Source: CAD feature listing. Evaluate the final solid. Frame: model axes, mm. Face numbers are marked on the shaded views. Coordinates: 2 decimals unless noted, no trailing zeros. Write each loop counter-clockwise with the first axis right and the second up, starting at its lowest first coordinate (ties: lowest second). Pieces come first, ordered by that corner, then holes. Notation, with made-up numbers: M 56,68.25 L 113,68.25 A15 cw 113,75.25 Z; hole C 33,-39.5 d11. An arc over 180 degrees is marked long. One line per item, written item: value. Start each with the question number.
Item 1: Mould query, pull axis Y, two halves, no side actions, for the marked faces 1 and 2. Classes: released by +Y, released by -Y, zero draft, split by the parting line, or undercut.
Item 2: Ray query, L1, parallel to Y at x = 73, z = 2.5; L2, parallel to Y at x = 50, z = 3.75; L3, parallel to Y at x = 81.5, z = 2. Return the intervals inside material, ascending. Write a range as from..to.
Item 3: Pin query (flat end, axial travel): P1, Ø1.5, axis at x = 123.5, z = 1.5, coming from the +Y side; P2, Ø5, axis at x = 86.035, y = -31.25, coming from the -Z side; P3, Ø20, axis at x = 59.509, y = 0, coming from the +Z side; P4, Ø4, axis at x = 39.549, y = 67.25, coming from the -Z side. Return the tip coordinate at first contact, or that it passes through.
Item 4: Cut plane A-A, the plane y = 0. Output: boundary loops of the cut face in (x, z), then the cut area to 3 significant figures.
Item 5: Cut plane D-D, the plane y = 40.5. Output: boundary loops of the cut face in (x, z), then the cut area to 3 significant figures.
Item 6: Cut plane C-C, the plane y = -23.5. Output: boundary loops of the cut face in (x, z), then the cut area to 3 significant figures.
Item 7: Cut plane B-B, the plane y = 67.25. Output: boundary loops of the cut face in (x, z).
Autodesk Inventor part; units mm, degrees
ref_plane "YZ Plane" through (0, 0, 0) normal (1, 0, 0) x (0, 1, 0)
ref_plane "XZ Plane" through (0, 0, 0) normal (0, 1, 0) x (-1, 0, 0)
ref_plane "XY Plane" through (0, 0, 0) normal (0, 0, 1) x (1, 0, 0)
sketch "Sketch1" plane through (0, 0, 0) normal (0, 0, 1) x (1, 0, 0)
  circle A0 centre (-11.3135, -11.3135) radius 2
  circle A1 centre (-11.3135, 11.3135) radius 2
  circle A2 centre (11.3135, 11.3135) radius 2
  circle A3 centre (11.3135, -11.3135) radius 2
  circle A4 centre (-15.3135, 11.3135) radius 2
  circle A5 centre (-7.3135, 11.3135) radius 2
  circle A6 centre (7.3135, 11.3135) radius 2
  circle A7 centre (15.3135, 11.3135) radius 2
  circle A8 centre (15.3135, -11.3135) radius 2
  circle A9 centre (7.3135, -11.3135) radius 2
  circle A10 centre (-7.3135, -11.3135) radius 2
  circle A11 centre (-15.3135, -11.3135) radius 2
  line L0 (-15.3135, 13.3135) -> (-7.3135, 13.3135)
  line L1 (-7.3135, 9.3135) -> (-15.3135, 9.3135)
  line L2 (-15.3135, -9.3135) -> (-7.3135, -9.3135)
  line L3 (-7.3135, -13.3135) -> (-15.3135, -13.3135)
  line L4 (7.3135, -9.3135) -> (15.3135, -9.3135)
  line L5 (15.3135, -13.3135) -> (7.3135, -13.3135)
  line L6 (15.3135, 9.3135) -> (7.3135, 9.3135)
  line L7 (15.3135, 13.3135) -> (7.3135, 13.3135)
  circle A12 centre (0, 0) radius 8.25
  circle A13 centre (5, 0) radius 8.25
  circle A14 centre (-5, 0) radius 8.25
  line L8 (-5, 8.25) -> (5, 8.25)
  line L9 (5, -8.25) -> (-5, -8.25)
  circle A15 centre (0, 0) radius 42.5
  circle A16 centre (59.509, 0) radius 50.7821
  line L10 (-5.9149, 42.0864) -> (52.4415, 50.2878)
  line L11 (-5.9149, -42.0864) -> (52.4415, -50.2878)
  line L12 (-13.25, 0) -> (13.25, 0)
  circle A17 centre (59.509, 0) radius 11
  arc A18 (-5.9149, 42.0864) -> (-5.9149, -42.0864) centre (0, 0) ccw
  line L13 (-42.5, 0) -> (156.5802, 0)
  circle A19 centre (59.509, 0) radius 90
  point P0 (-3.1314, -32.3793)
  point P1 (23.2633, -35.5678)
  point P2 (23.2633, 35.5678)
  point P3 (-2.5, -7.8621)
  point P4 (0, -8.25)
  dimension "d0" = 4
  dimension "d1" = 22.627
  dimension "d2" = 22.627
  dimension "d3" = 11.3135
  dimension "d4" = 11.3135
  dimension "d5" = 4
  dimension "d6" = 4
  dimension "d7" = 4
  dimension "d8" = 4
  dimension "d9" = 4
  dimension "d10" = 4
  dimension "d11" = 4
  dimension "d12" = 4
  dimension "d15" = 16.5
  dimension "d16" = 5
  dimension "d17" = 5
  dimension "d18" = 85
  dimension "d19" = 8
  dimension "d20" = 59.509
  dimension "d21" = 22
  dimension "d24" = 85
  dimension "d116" = 180
extrude "Extrusion1" add sketch "Sketch1" along normal blind 10 contours A0 | A10 L3 A0 | A0 L2 A10 | A10 | A0 A11 L2 | L3 A11 A0 | A11 | A1 | A5 L1 A1 | A1 L0 A5 | A5 | A1 A4 L0 | L1 A4 A1 | A4 | A2 A16 | A7 L6 A2 | A2 L7 A7 | A7 | L7 A16 A15 L13 A13 L6 A7 | A2 A16 L7 | L6 A16 A2 | A16 A2 | A2 A6 L7 A16 | L7 A6 L6 A16 A13 L8 A14 L13 A19 A15 | A16 L6 A6 A2 | A6 | A16 L13 A17 A15 | A15 L10 A16 | A16 L12 A12 A13 | A13 L12 A16 | L13 A17 A16 A15 | A15 A16 L5 A8 L4 A13 L13 | A15 A19 L13 A16 L10 | A13 A16 L12 | A13 A12 L8 | A16 A13 A12 L12 | A16 L11 A15 | A15 A19 L13 A14 L9 A13 A16 L4 A9 L5 | L13 A19 A15 L11 A16 | A13 A14 A12 | A12 L12 A14 A13 | A12 A14 L8 | A12 A13 A14 L12 | A16 A3 L5 | L5 A9 A3 A16 | L9 A12 A13 | A16 A3 A9 L4 | L4 A3 A16 | A14 L12 A13 | A13 L12 A12 A14 | A12 L12 A14 | A12 A14 A13 | A14 A13 L12 | A3 A16 | A3 A8 L5 | A9 | A3 A16 | L12 A12 A14 | L9 A14 A12 | L4 A8 A3 | A13 A14 A12 L12 | A8
sketch "Sketch18" plane through (59.509, 0, 0) normal (0, 0, -1) x (-1, 0, 0)
  circle A0 centre (0, 0) radius 35
  circle A1 centre (0, 0) radius 90
  circle A2 centre (0, 0) radius 11
  circle A3 centre (0, 0) radius 16
  point P0 (59.509, 0)
  dimension "d127" = 70
  dimension "d130" = 5
extrude "Extrusion9" cut sketch "Sketch18" against normal blind 6.5 contours A0 | A2
sketch "Sketch20" plane through (59.509, 0, 0) normal (0, 0, -1) x (-1, 0, 0)
  circle A0 centre (0, 0) radius 11
  circle A1 centre (0, 0) radius 11
  circle A2 centre (0, 0) radius 6
  point P0 (59.509, 0)
  dimension "d136" = 12
extrude "Extrusion11" add sketch "Sketch20" against normal blind 3
sketch "Sketch22" plane through (59.509, 0, 0) normal (0, 0, -1) x (-1, 0, 0)
  circle A0 centre (55.7915, 31.25) radius 1.621
  circle A1 centre (71.5915, 31.25) radius 1.621
  circle A2 centre (71.5915, -31.2504) radius 1.621
  circle A3 centre (55.7915, -31.2504) radius 1.621
  circle A4 centre (71.5915, -31.2504) radius 1.621
  circle A5 centre (55.7915, -31.2504) radius 1.621
  circle A6 centre (71.5915, 31.25) radius 1.621
  circle A7 centre (55.7915, 31.25) radius 1.621
  point P0 (59.509, 0)
hole "Hole4" at (-12.0825, 31.25, 0) at (3.7175, 31.25, 0) at (-12.0825, -31.2504, 0) at (3.7175, -31.2504, 0) direction (0, 0, 1) diameter 4.2 end through all countersink diameter 9.4 countersink angle 90
sketch "Sketch23" plane through (59.509, 0, 0) normal (0, 0, -1) x (-1, 0, 0)
  circle A0 centre (-26.526, -31.25) radius 2.4585
  circle A1 centre (26.526, -31.25) radius 2.4585
  circle A2 centre (-26.526, 31.25) radius 1.621
  circle A3 centre (26.526, 31.25) radius 1.621
  circle A4 centre (26.526, -31.25) radius 2.4585
  circle A5 centre (26.526, 31.25) radius 1.621
  circle A6 centre (-26.526, -31.25) radius 2.4585
  circle A7 centre (0, 0) radius 90
  circle A8 centre (0, 0) radius 11
  circle A9 centre (-26.526, 31.25) radius 1.621
  point P0 (59.509, 0)
hole "Hole5" at (86.035, 31.25, 0) at (86.035, -31.25, 0) at (32.983, -31.25, 0) at (32.983, 31.25, 0) direction (0, 0, 1) diameter 4.5 depth 14.2 tip angle 118 countersink diameter 9.4 countersink angle 90
sketch "Sketch24" plane through (59.509, 0, 0) normal (0, 0, -1) x (-1, 0, 0)
  circle A0 centre (-19.96, 67.25) radius 1.621
  circle A1 centre (19.96, 67.25) radius 1.621
  circle A2 centre (-19.96, 67.25) radius 2.1
  circle A3 centre (19.96, 67.25) radius 2.1
  point P0 (59.509, 0)
  dimension "d152" = 4.2
  dimension "d153" = 4.2
hole "Hole6" at (79.469, 67.25, 0) at (39.549, 67.25, 0) direction (0, 0, 1) diameter 4.5 depth 15 tip angle 118 countersink diameter 9.4 countersink angle 90
equation "\"d2\" = d1"
equation "\"d5\" = d0"
equation "\"d6\" = d5"
equation "\"d7\" = d6"
equation "\"d8\" = d7"
equation "\"d9\" = d5"
equation "\"d10\" = d9"
equation "\"d11\" = d10"
equation "\"d12\" = d11"
equation "\"d17\" = d16"
properties part number "base bovenkant v2" material "Aluminum 6061"
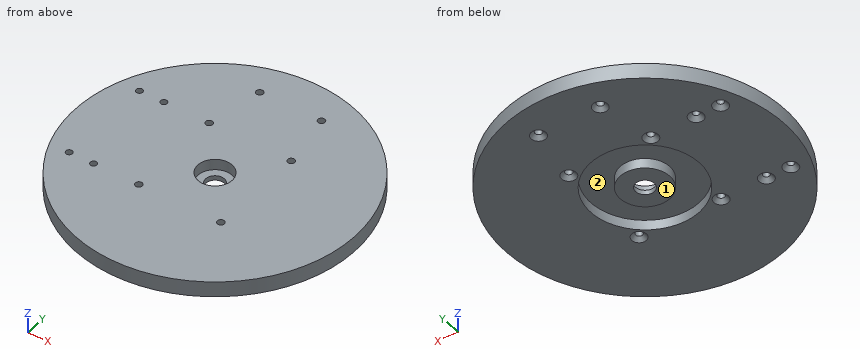
From the geometry:
1. face 1: zero draft
1. face 2: undercut
2. L1: y = -88.98..-32.3, -8.6..8.6, 32.3..88.98
2. L2: y = -89.5..-33.68, -12.87..-5.53, 5.53..12.87, 33.68..89.5
2. L3: y = -87.27..-27.23, 27.23..65.47, 69.03..87.27
3. P1: stops at y = 64.04
3. P2: stops at z = 2.2
3. P3: stops at z = 3
3. P4: passes through
4. outline: M -30.49,0 L 24.51,0 L 24.51,6.5 L 43.51,6.5 L 43.51,0 L 53.51,0 L 53.51,3 L 48.51,3 L 48.51,10 L -30.49,10 Z; M 65.51,0 L 75.51,0 L 75.51,6.5 L 94.51,6.5 L 94.51,0 L 149.51,0 L 149.51,10 L 70.51,10 L 70.51,3 L 65.51,3 Z
4. area: 1,360 mm²
5. outline: M -20.86,0 L 139.88,0 L 139.88,10 L -20.86,10 Z
5. area: 1,610 mm²
6. outline: M -27.37,0 L 33.57,0 L 33.57,6.5 L 85.45,6.5 L 85.45,0 L 146.39,0 L 146.39,10 L -27.37,10 Z
6. area: 1,400 mm²
7. outline: M -0.3,0 L 34.85,0 L 37.3,2.45 L 37.3,10 L -0.3,10 Z; M 41.8,2.45 L 44.25,0 L 74.77,0 L 77.22,2.45 L 77.22,10 L 41.8,10 Z; M 81.72,2.45 L 84.17,0 L 119.32,0 L 119.32,10 L 81.72,10 Z
